Geometry check sheet. Reference: drawing and pictorial views, mm from the part's lowest x, y, z. A direction names the side the tool comes from. Give positions to 0.01 mm unless a question says otherwise; leave off trailing zeros. Write each loop counter-clockwise with the first axis right and the second up, starting at its lowest first coordinate (ties: lowest second). Pieces come first, ordered by that corner, then holes. Notation, with made-up numbers: (8.5, -8) -> (25.5, -8) arc R17 ccw to (25.5, 21) -> close; hole circle Ø11 at (-1.75, 6). An arc over 180 degrees is marked (long way). Write each question's results on one line, items separated by ' | '. Start each with the question number.
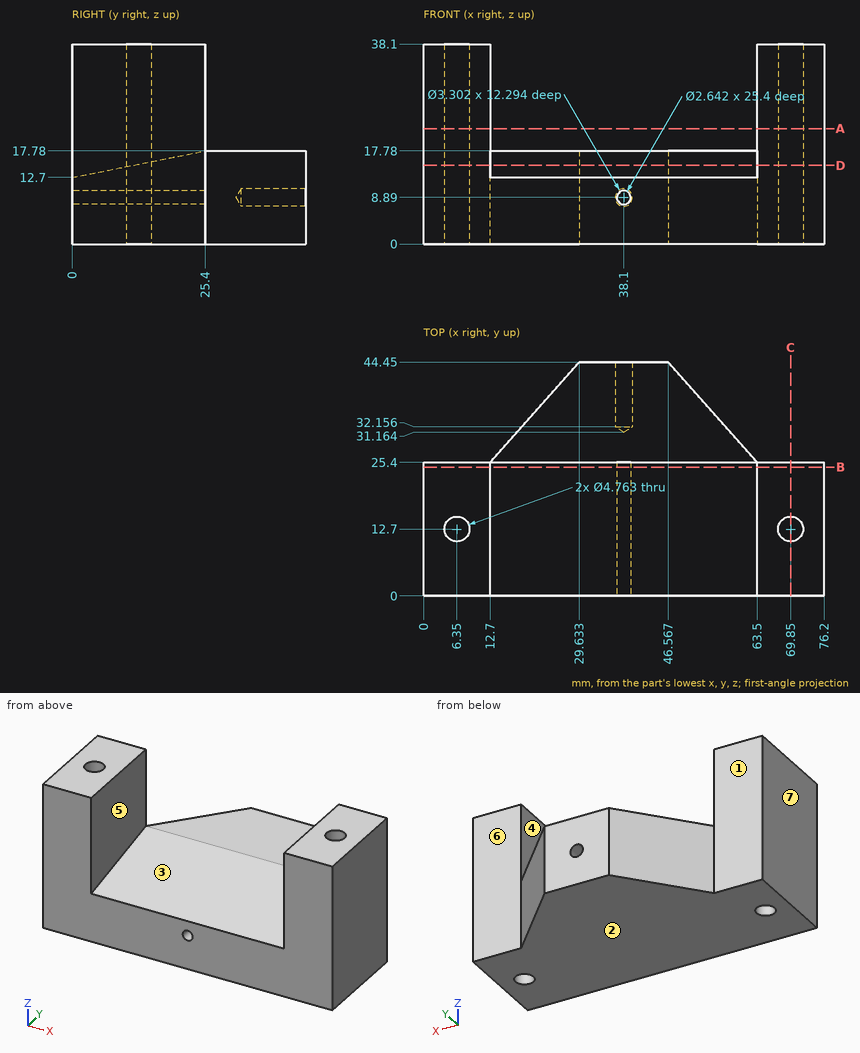
Item 1: Section check B-B on y = 24.5. Record the boundary of the cut face in (x, z), then the cut area to 3 significant figures.
Item 2: Set-up check for the marked faces 1, 2 and 3: record each of +Z, -Z, +X, -X, +Y, -Y from which the full face is reachable in a straight line by a thin tool's end or side.
Item 3: Mould release check, pull along X, two halves, no side actions. Record for the marked faces 4, 5, 6 and 7: pulls with the +X half, pulls with the -X half, needs draft (parallel to the pull), parting line crosses it, or undercut.
Item 4: Section check A-A on z = 22. Record the boundary of the cut face in (x, y).
Item 5: Section check D-D on z = 15. Record the boundary of the cut face in (x, y).
Item 6: Depth check by flat-ended pin: pin 1 Ø12 at (x, y) = (22.5, 38.5) entering from +Z; pin 2 Ø4.5 at (x, y) = (6.35, 12.7) entering from +Z; pin 3 Ø10 at (x, z) = (9.5, 19) entering from +Y (1 decimal); pin 4 Ø6 at (x, y) = (49.5, 8) entering from +Z. Enter the tip coordinate at first touch or a pass-through.
Item 7: Thickness scan on probe 1 along X at (y, z) = (20.5, 32); probe 2 along Z at (x, y) = (38.1, 37.5); probe 3 along X at (y, z) = (12, 25) (1 decimal). Record the ranges inside material, lowest first. Write a range as from..to.
Item 8: Section check C-C on x = 69.85. Record the boundary of the cut face in (y, z).
Check sheet entries:
1) outline: (0, 0) -> (76.2, 0) -> (76.2, 38.1) -> (63.5, 38.1) -> (63.5, 17.6) -> (12.7, 17.6) -> (12.7, 38.1) -> (0, 38.1) -> close; hole circle Ø2.64 at (38.1, 8.89) | area: 1,860 mm^2
2) face 1: +Z, -Z, -X, +Y | face 2: -Z, +X, -X, +Y, -Y | face 3: +Z, -Y
3) face 4: undercut | face 5: undercut | face 6: needs draft | face 7: pulls with the -X half
4) outline: (0, 0) -> (12.7, 0) -> (12.7, 25.4) -> (0, 25.4) -> close; (63.5, 0) -> (76.2, 0) -> (76.2, 25.4) -> (63.5, 25.4) -> close; hole circle Ø4.76 at (6.35, 12.7); hole circle Ø4.76 at (69.85, 12.7)
5) outline: (0, 0) -> (12.7, 0) -> (12.7, 11.5) -> (63.5, 11.5) -> (63.5, 0) -> (76.2, 0) -> (76.2, 25.4) -> (63.5, 25.4) -> (46.57, 44.45) -> (29.63, 44.45) -> (12.7, 25.4) -> (0, 25.4) -> close; hole circle Ø4.76 at (6.35, 12.7); hole circle Ø4.76 at (69.85, 12.7)
6) pin 1: stops at z = 17.78 | pin 2: passes through | pin 3: stops at y = 27.3 | pin 4: stops at z = 14.9
7) probe 1: x = 0..12.7, 63.5..76.2 | probe 2: z = 0..7.24, 10.54..17.78 | probe 3: x = 0..4.1, 8.6..12.7, 63.5..67.6, 72.1..76.2
8) outline: (0, 0) -> (10.32, 0) -> (10.32, 38.1) -> (0, 38.1) -> close; (15.08, 0) -> (25.4, 0) -> (25.4, 38.1) -> (15.08, 38.1) -> close
